Check sheet for the drawn part. Datum: minimum x, y, z corner. Units: mm. A direction names the side the tool comes from. Give positions to 0.01 mm unless a question says otherwise; leave off trailing zeros. Write each loop counter-clockwise with the first axis right and the second up, starting at its lowest first coordinate (ties: lowest second). Pieces come first, ordered by that corner, then holes. Notation, with made-up numbers: (66, -33.75) -> (80, -33.75) arc R20 cw to (80, 5.25) -> close; hole circle Ø3 at (-40, 45). An arc over 180 degrees is marked (long way). Write item = value, one per line. Start each with the question number.
1. Thickness scan on line 1 along Y through (x, z) = (5, 2.8); line 2 along Y through (x, z) = (5, 1.75); line 3 along Z through (x, y) = (6.5, 8.25). Record the ranges inside material, lowest first.
2. Set-up check for the marked faces 1, 2 and 3: record each of +Z, -Z, +X, -X, +Y, -Y from which the full face is reachable in a straight line by a thin tool's end or side.
3. Cross-section at A-A, the plane y = 5. Record the cut outline in (x, z), plus the area to 3 significant figures.
4. Cross-section at C-C, the plane z = 5.1. Record the cut outline in (x, y), plus the area to 3 significant figures.
5. Cross-section at D-D, the plane y = 1. Record the cut outline in (x, z).
6. Depth check by flat-ended pin: P1, Ø1, axis at x = 3.5, y = 8, coming from the +Z side; P2, Ø2, axis at x = 1, z = 2.5, coming from the +Y side; P3, Ø3, axis at x = 1.5, z = 2, coming from the +Y side. Enter the tip coordinate at first touch or a pass-through.
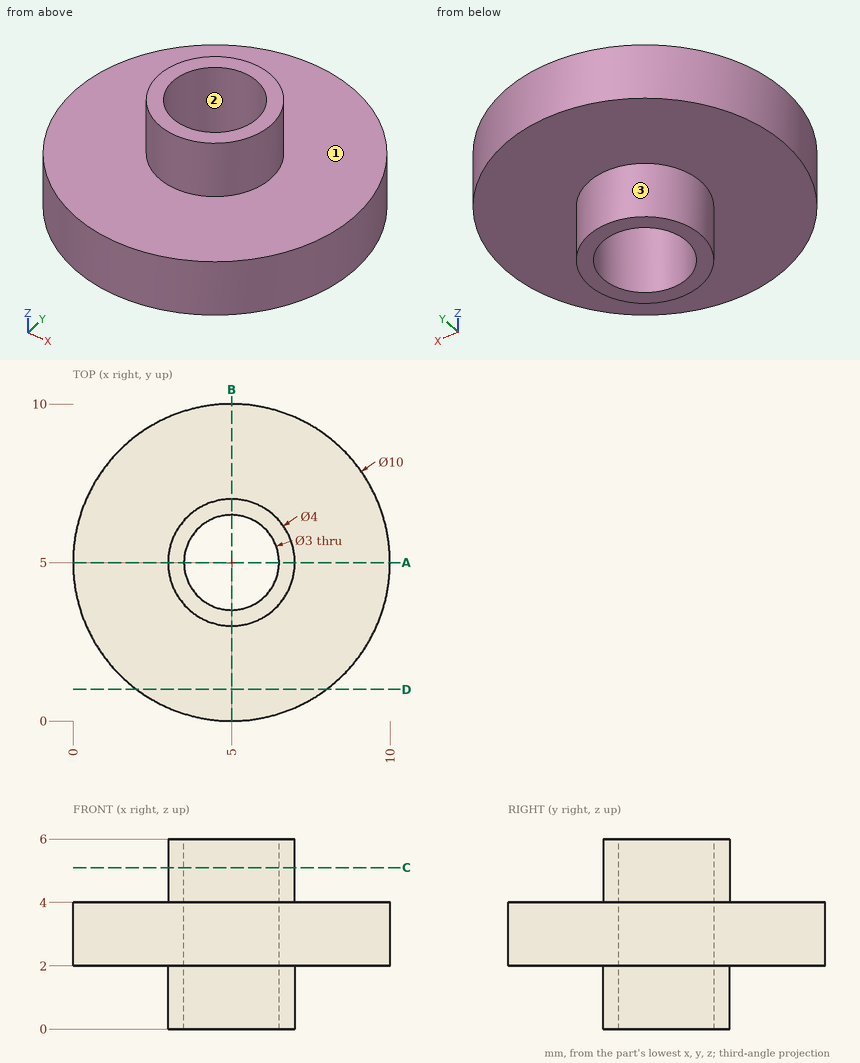
Answers:
q1.line_1 = 0 to 3.5, 6.5 to 10
q1.line_2 = 3 to 3.5, 6.5 to 7
q1.line_3 = 2 to 4
q2.face_1 = +Z
q2.face_2 = +Z, -Z
q2.face_3 = -Z
q3.outline = (0, 2) -> (3, 2) -> (3, 0) -> (3.5, 0) -> (3.5, 6) -> (3, 6) -> (3, 4) -> (0, 4) -> close; (6.5, 0) -> (7, 0) -> (7, 2) -> (10, 2) -> (10, 4) -> (7, 4) -> (7, 6) -> (6.5, 6) -> close
q3.area = 18.0 mm^2
q4.outline = circle Ø4 at (5, 5); hole circle Ø3 at (5, 5)
q4.area = 5.50 mm^2
q5.outline = (2, 2) -> (8, 2) -> (8, 4) -> (2, 4) -> close
q6.P1 = 4
q6.P2 = 9
q6.P3 = 9.58
